Could you check a few things on this model? Use its own coordinates, in mm. Round coordinates to 2 decimals unless told otherwise and drop trailing zeros. Write each loop counter-clockwise with the first axis right and the second up, starting at its lowest first coordinate (ties: lowest second). Pieces come first, ordered by that corner, then holes. Notation, with made-up numbers: M 31,8.5 L 85,8.5 A27 ccw 85,32.5 Z; hole C 13,23 d11. An arc over 180 degrees is marked long. One line per item, written item: value. Start each with the question number.
(1) I want a section at C-C on z = 29. Please give me the cut outline in (x, y).
(2) I'm going to push flat-ended pins straight in: pin 1 Ø3 at (y, z) = (4, 29.5) entering from -X; pin 2 Ø6 at (x, z) = (-4, 14) entering from -Y; pin 3 Ø4 at (x, z) = (3.5, 28.5) entering from +Y; pin 4 Ø3 at (x, y) = (0, 0) entering from +Z. Where does each tip first touch, or does it pass through?
(3) If I drill on L1, parallel to Y at x = 0, z = 30.25; L2, parallel to Y at x = 0, z = 15.5; L3, parallel to X at y = 2.25, z = 3.5, over which ranges is the centre line in solid material (lowest first)?
(4) I want a section at D-D on z = 16. Please give me the cut outline in (x, y).
(5) Thinking about a two-plate mould opening in Y: for faces 1 (the face through (1.617, -0.67, 9.924)), 2 (the face through (-1.73, 7.81, 17.26)), 3 (the face through (-0.738, -2.345, 27.395)), 4 (the face through (0, 2, 0)), which applies, released by +Y, released by -Y, zero draft, split by the parting line, or undercut?
(6) I want a section at A-A on y = 0. Please give me the cut outline in (x, z), and give its area (3 significant figures).
Solid Edge part; units mm, degrees
sketch "Sketch1" plane through (0, 0, 0) normal (0, 0, 1) x (1, 0, 0)
  circle A0 centre (0, 0) radius 8
extrude "Protrusion1" add sketch "Sketch1" along normal blind 35
sketch "Sketch2" plane through (0, 0, 35) normal (0, 0, 1) x (1, 0, 0)
  circle A0 centre (0, 0) radius 1.75
extrude "Cutout1" cut sketch "Sketch2" against normal through all
hole "Hole_1" at (0, 0, 35) direction (0, 0, -1) diameter 4.917 depth 15 tip angle 118 thread major 6 thread length 15
extrude "Cutout2" [suppressed]
properties material "Polyurethene"
Found:
1. outline: C 0,0 d16; hole C 0,0 d4.92
2. pin 1: stops at x = -7.6
2. pin 2: stops at y = -7.94
2. pin 3: stops at y = 7.86
2. pin 4: passes through
3. L1: y = -8 to -2.46, 2.46 to 8
3. L2: y = -8 to -1.75, 1.75 to 8
3. L3: x = -7.68 to 7.68
4. outline: C 0,0 d16; hole C 0,0 d3.5
5. face 1: undercut
5. face 2: split by the parting line
5. face 3: undercut
5. face 4: zero draft
6. outline: M -8,0 L -1.75,0 L -1.75,19.57 L -2.46,20 L -2.46,35 L -8,35 Z; M 1.75,0 L 8,0 L 8,35 L 2.46,35 L 2.46,20 L 1.75,19.57 Z
6. area: 416 mm²
